Verification items for the finished model (mm, model axes). A direction names the side the tool comes from. Coordinates: 2 decimals unless noted, no trailing zeros. Order: outer loops, then holes, each group sorted by start corner. A loop starts at its lowest first (then second) coordinate and runs counter-clockwise, first axis right, second up. Notation, with made-up numbers: M 84.5,0.25 L 109.5,0.25 A17 cw 109.5,13.25 Z; hole C 40,66.25 d3. An arc over 180 degrees is marked long. Return JSON: item names as keys, results as strings.
Solid Edge part; units mm, degrees
sketch "Sketch1" plane through (0, 0, 0) normal (0, 0, 1) x (1, 0, 0)
  line L0 (160, 0) -> (160, 40)
  line L1 (160, 40) -> (0, 40)
  line L2 (0, 40) -> (0, 0)
  line L3 (0, 0) -> (160, 0)
extrude "Protrusion1" add sketch "Sketch1" along normal blind 5
sketch "Sketch2" plane through (75, 20, 5) normal (0, 0, 1) x (1, 0, 0)
  line L0 (80, 10) -> (85, 10)
  line L1 (85, 10) -> (85, -10)
  line L2 (85, -10) -> (80, -10)
  line L3 (80, -10) -> (80, 10)
  line L4 (-70, -10) -> (-70, 10)
  line L5 (-70, 10) -> (-75, 10)
  line L6 (-75, 10) -> (-75, -10)
  line L7 (-75, -10) -> (-70, -10)
extrude "ExtrudedProtrusion_2" add sketch "Sketch2" along normal blind 70
hole "Bohrung_1" at (20, 30, 5) direction (0, 0, -1) diameter 4.2 end up to next start chamfer 1 start chamfer angle 45
hole "Hole1" at (20, 10, 5) direction (0, 0, -1) diameter 4.2 end up to next start chamfer 1 start chamfer angle 45
hole "Hole2" at (140, 10, 5) direction (0, 0, -1) diameter 4.2 end up to next start chamfer 1 start chamfer angle 45
hole "Hole3" at (140, 30, 5) direction (0, 0, -1) diameter 4.2 end up to next start chamfer 1 start chamfer angle 45
hole "Bohrung_6" at (160, 20, 55) direction (-1, 0, 0) diameter 10 end through all
Q1. Cross-section at D-D, the plane z = 8. Record the boundary of the cut face in (x, y).
Values:
{"outline": "M 0,10 L 5,10 L 5,30 L 0,30 Z; M 155,10 L 160,10 L 160,30 L 155,30 Z"}
Q2. Cross-section at C-C, the plane x = 20. Record the boundary of the cut face in (y, z).
Values:
{"outline": "M 0,0 L 7.9,0 L 7.9,4 L 6.9,5 L 0,5 Z; M 12.1,0 L 27.9,0 L 27.9,4 L 26.9,5 L 13.1,5 L 12.1,4 Z; M 32.1,0 L 40,0 L 40,5 L 33.1,5 L 32.1,4 Z"}
Q3. Draft check along Z on faces 1 (the face through (158, 17, 59)), 2 (the face through (158, 20, 75)), 3 (the face through (160, 20, 37)). Enter one of: pulls with the +Z half, pulls with the -Z half, needs draft (parallel to the pull), parting line crosses it, or undercut.
Values:
{"face 1": "undercut", "face 2": "pulls with the +Z half", "face 3": "needs draft"}
Q4. Cross-section at B-B, the plane z = 52. Record the boundary of the cut face in (x, y), and give its area (3 significant figures).
Values:
{"outline": "M 0,10 L 5,10 L 5,16 L 0,16 Z; M 0,24 L 5,24 L 5,30 L 0,30 Z; M 155,10 L 160,10 L 160,16 L 155,16 Z; M 155,24 L 160,24 L 160,30 L 155,30 Z", "area": "120 mm^2"}
Q5. Go/stop test with flat-tipped pins: pin 1 (4 mm diameter, centred on x = 1.5, z = 37.5, fed in from -Y); pin 2 (10 mm diameter, centred on x = 86.5, y = 16, fed in from +Z); pin 3 (2.5 mm diameter, centred on x = 2.5, z = 56.5, fed in from +Y). Record where each tip stops, or that it passes through.
Values:
{"pin 1": "y = 10", "pin 2": "z = 5", "pin 3": "y = 30"}
Q6. Cross-section at A-A, the plane y = 17. Record the boundary of the cut face in (x, z).
Values:
{"outline": "M 0,0 L 160,0 L 160,51 L 155,51 L 155,5 L 5,5 L 5,51 L 0,51 Z; M 0,59 L 5,59 L 5,75 L 0,75 Z; M 155,59 L 160,59 L 160,75 L 155,75 Z"}
Q7. Tool access check on faces 4 (the face through (157, 30, 40)), 5 (the face through (155, 20, 40)), 6 (the face through (0, 20, 37)), 7 (the face through (158, 10, 40)), 8 (the face through (3, 17, 59)). Record the directions out of +Z, -Z, +X, -X, +Y, -Y that give a thin tool (end or side, any length) a straight path to the whole face; none if there is none.
Values:
{"face 4": "+Z, +X, -X, +Y", "face 5": "+Z, +Y, -Y", "face 6": "+Z, -Z, -X, +Y, -Y", "face 7": "+Z, +X, -X, -Y", "face 8": "+X, -X"}
Q8. Material ranges on line 1 along X through (y, z) = (30, 1.15); line 2 along Y through (x, z) = (140, 1.1); line 3 along X through (y, z) = (25, 39), recorded low to high.
Values:
{"line 1": "0 to 17.9, 22.1 to 137.9, 142.1 to 160", "line 2": "0 to 7.9, 12.1 to 27.9, 32.1 to 40", "line 3": "0 to 5, 155 to 160"}
